The figure shows three views and two pictorial views of one solid part (mm, origin at its lowest corner). Answer the questions. Give positions to 0.01 mm unless a question says otherwise; leave off trailing zeros. Order: outer loops, then holes, each group sorted by start corner. A loop starts at its lowest first (then second) coordinate and runs counter-clockwise, first axis right, second up. Notation, with made-up numbers: M 84,-39 L 92,-39 A21 ccw 92,-22 Z; hole C 3,52.5 d2. An arc over 180 degrees is marked long. Answer as a JSON object with one key per item and string values. Group by question number.
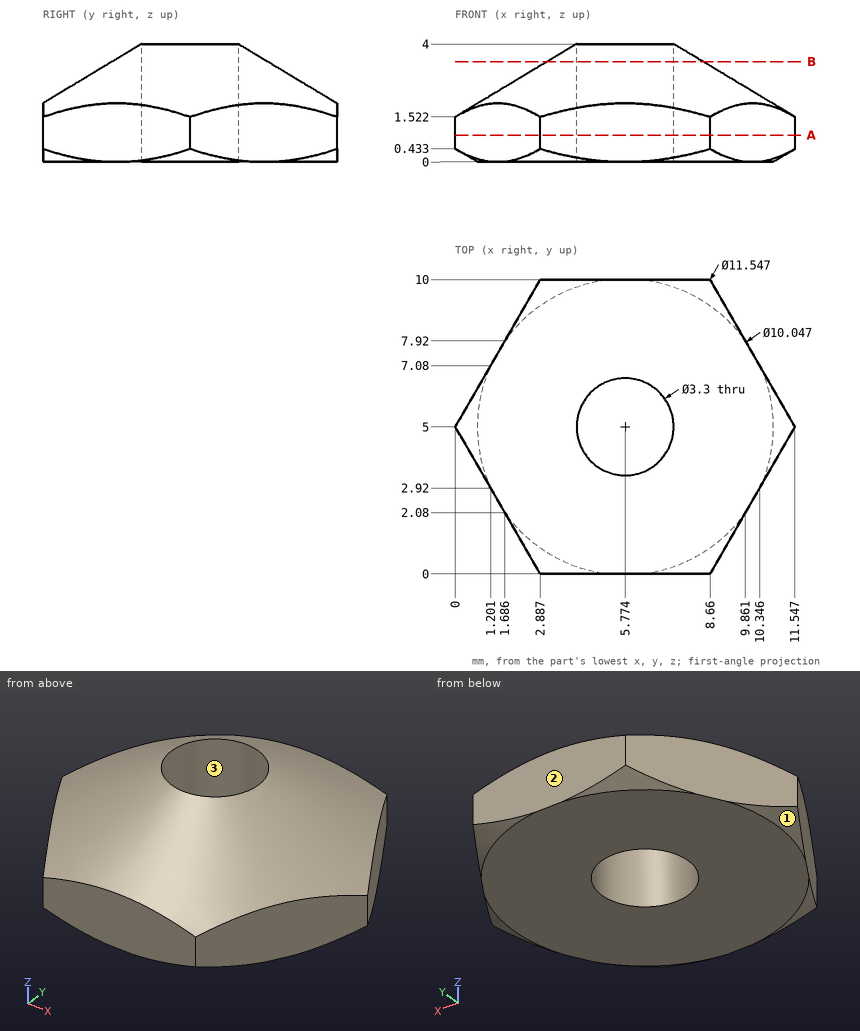
Item 1: Flat-ended cylindrical pins translate along their axes: P1, Ø4.5, axis at x = 5.77, y = 5, coming from the +Z side; P2, Ø4, axis at x = 7.5, y = 1.5, coming from the +Z side. Find the tip coordinate at first contact, or state that the pin passes through.
Item 2: Section A-A (z = 0.9) is taken. Determine the outline of the cut face in (x, y).
Item 3: Determine the mould class of the marked faces 1, 2 and 3 for opening direction Y: released by +Y, released by -Y, zero draft, split by the parting line, or undercut.
Item 4: Consider probe 1 along Y at (x, z) = (5.25, 2.25) (1 decimal); probe 2 along Y at (x, z) = (7.25, 3.7) (1 decimal); probe 3 along X at (y, z) = (6, 0.55) (1 decimal). Determine where each line is inside the solid, lowest interval first. Write a range as from..to.
Item 5: Section B-B (z = 3.4) is taken. Determine the outline of the cut face in (x, y), and give its area (3 significant figures).
Values found:
{
 "1": {"P1": "stops at z = 4", "P2": "stops at z = 3.85"},
 "2": {"outline": "M 0,5 L 2.89,0 L 8.66,0 L 11.55,5 L 8.66,10 L 2.89,10 Z; hole C 5.77,5 d3.3"},
 "3": {"face 1": "split by the parting line", "face 2": "released by +Y", "face 3": "undercut"},
 "4": {"probe 1": "y = 0.5..3.4, 6.6..9.5", "probe 2": "y = 3.4..4.3, 5.7..6.6", "probe 3": "x = 0.6..4.5, 7.1..11"},
 "5": {"outline": "C 5.77,5 d5.3; hole C 5.77,5 d3.3", "area": "13.5 mm^2"}
}
